The listing builds one solid part. Answer for the finished solid, in the listing's coordinates (mm). A direction names the side the tool comes from. Round coordinates to 2 decimals unless told otherwise and drop trailing zeros. Order: outer loops, then holes, each group sorted by start corner. A loop starts at its lowest first (then second) coordinate and runs counter-clockwise, first axis right, second up. Notation, with made-up numbers: (9.25, 71.25) - (21.25, 71.25) arc R11 cw to (21.25, 77.25) - close; hole circle Ø11 at (9, 48.25). An arc over 180 degrees is marked (long way). Use CSV: the item, a comma, the result in double quotes. Start each with the question number.
Item 1: Determine the mould class of faces 6 (the flat face through (0, 5, 68)), 7 (the cylindrical face through (9.87, 27.62, 43.83)), 8 (the flat face through (13.05, 24, 51)), 9 (the flat face through (-0.183, 19.859, 57.263)) for opening direction Y: +Y half, -Y half, draft (parallel to the pull), parting line (faces both ways), or undercut.
Item 2: Find section A-A, the plane x = -1. Give the vertices of the cut face in (y, z).
Item 3: Flat-ended cylindrical pins translate along their axes: P1, Ø1, axis at x = -12, z = 64.5, coming from the +Y side; P2, Ø4, axis at x = 1.5, z = 68.5, coming from the -Y side; P3, Ø6, axis at x = 9.5, y = 28.5, coming from the +Z side. Find the tip coordinate at first contact, or state that the pin passes through.
Item 4: For faces 1 (the flat face through (-20, 0, 65)), 2 (the flat face through (-0.183, 27.359, 44.273)), 3 (the flat face through (0.41, 26.28, 43.1)), 4 (the cylindrical face through (9.59, 17.09, 62.06)), 5 (the flat face through (-10, 2, 68)), determine the directions among +Z, -Z, +X, -X, +Y, -Y from which every point of the face is accessible in a straight line to the end or side of a thin tool.
Item 5: Find section D-D, the plane x = -16. Give the vertices of the cut face in (y, z), plus the area to 3 significant figures.
Item 6: Find section B-B, the plane y = 23.5. Give the vertices of the cut face in (x, z), plus the area to 3 significant figures.
Item 7: Find section C-C, the plane z = 54.5. Give the vertices of the cut face in (x, y), plus the area to 3 significant figures.
Item 8: Straight lines are drawn through the part: line 1 along Y through (x, z) = (-3, 67); line 2 along Y through (x, z) = (-4, 40); line 3 along Z through (x, y) = (13, 8). For each, find the intervals that lie inside material, in ascending order. Write a range as [from, to].
```python
from build123d import *

# Parameters (mm, degrees)
BOSS_EXTRUDE1_DEPTH     = 18
BOSS_EXTRUDE2_DEPTH     = 3
CUT_EXTRUDE3_DEPTH      = 84.253650708
CUT_EXTRUDE3_DEPTH_BACK = 84.253650708
CUT_EXTRUDE4_DEPTH      = 84.253650708
SKETCH5_R               = 1.25
SKETCH5_W               = 26.1
SKETCH5_H               = 15
CUT_EXTRUDE1_DEPTH      = 7
SKETCH6_W               = 20
SKETCH6_H               = 10
CUT_EXTRUDE2_DEPTH      = 84.253650708


with BuildPart() as part:
    # Sketch1 → Boss-Extrude1 (new body)
    with BuildSketch(Plane(origin=(0, 0, 0), x_dir=(1, 0, 0), z_dir=(0, 1, 0))):
        with BuildLine():
            Line((-29.583278322, -63.441545093), (-29.583278322, -60.115136561))
            ThreePointArc((-29.583278322, -60.115136561), (0, -67), (29.583278322, -60.115136561))
            Line((29.583278322, -60.115136561), (29.583278322, -63.441545093))
            ThreePointArc((29.583278322, -63.441545093), (0, -70), (-29.583278322, -63.441545093))
        make_face()
    extrude(amount=BOSS_EXTRUDE1_DEPTH)

    # Sketch3 → Boss-Extrude2 (add)
    with BuildSketch(Plane(origin=(0, 40.970994853, 23.654614907), x_dir=(-1, 0, 0), z_dir=(-1.9937140685199517e-15, -0.8660254037844395, -0.49999999999999856))):
        Polygon((29.583278322, -45.941989705), (29.583278322, -13.941989705), (-29.583278322, -13.941989705), (-29.583278322, -45.941989705), (-29.583278322, -53.515041118), (29.583278322, -53.515041118), align=None)
    extrude(amount=BOSS_EXTRUDE2_DEPTH)

    # Sketch7 → Cut-Extrude3 (cut, two sides: drawn at the far end of the back side and taken through both)
    with BuildSketch(Plane(origin=(0, 0, 0), x_dir=(0, 0, -1), z_dir=(1, 0, 0)).offset(-CUT_EXTRUDE3_DEPTH_BACK)):
        Polygon((-70, 14.213474294), (-63.441545093, 18), (-70, 18), align=None)
    extrude(amount=CUT_EXTRUDE3_DEPTH + CUT_EXTRUDE3_DEPTH_BACK, mode=Mode.SUBTRACT)

    # Sketch8 → Cut-Extrude4 (cut, through all)
    with BuildSketch(Plane.XZ):
        with BuildLine():
            Line((-29.583278322, 63.441545093), (-29.583278322, 71.549825609))
            Line((-29.583278322, 71.549825609), (29.583278322, 71.549825609))
            Line((29.583278322, 71.549825609), (29.583278322, 63.441545093))
            ThreePointArc((29.583278322, 63.441545093), (0, 70), (-29.583278322, 63.441545093))
        make_face()
    extrude(amount=-CUT_EXTRUDE4_DEPTH, mode=Mode.SUBTRACT)

    # Sketch5 → Cut-Extrude1 (cut)
    with BuildSketch(Plane(origin=(0, 40.970994853, 23.654614907), x_dir=(1, 0, 0), z_dir=(2.0433685445882858e-15, 0.8660254037844395, 0.49999999999999845))):
        with Locations(Location((-10.35, -22.991989705, 0), (0, 0, 270))):
            Circle(SKETCH5_R)
        with Locations(Location((10.35, -22.991989705, 0), (0, 0, 270))):
            Circle(SKETCH5_R)
        with Locations(Location((10.35, -46.191989705, 0), (0, 0, 270))):
            Circle(SKETCH5_R)
        with Locations(Location((-10.35, -46.191989705, 0), (0, 0, 270))):
            Circle(SKETCH5_R)
        with Locations((0, -32.161989705)):
            Rectangle(SKETCH5_W, SKETCH5_H)
    extrude(amount=-CUT_EXTRUDE1_DEPTH, mode=Mode.SUBTRACT)

    # Sketch6 → Cut-Extrude2 (cut, through all)
    with BuildSketch(Plane.XY):
        Rectangle(SKETCH6_W, SKETCH6_H)
    extrude(amount=CUT_EXTRUDE2_DEPTH, mode=Mode.SUBTRACT)


solid = part.part
```
Worked out:
1,face 6,"-Y half"
1,face 7,"undercut"
1,face 8,"draft"
1,face 9,"+Y half"
2,outline,"(5, 66.99) - (12.49, 66.99) - (18.54, 56.5) - (21.14, 58) - (14.22, 69.99) - (5, 69.99) - close; (26.04, 43.51) - (31.4, 34.23) - (34, 35.73) - (28.64, 45.01) - close"
3,P1,"stops at y = 17.68"
3,P2,"stops at y = 5"
3,P3,"stops at z = 45.01"
4,face 1,"+Z, -Z, +X, -X, -Y"
4,face 2,"+Z, -Y"
4,face 3,"-Z, -Y"
4,face 4,"none"
4,face 5,"+Z, -Z, -Y"
5,outline,"(0, 65.06) - (13.6, 65.06) - (31.4, 34.23) - (34, 35.73) - (15.28, 68.15) - (0, 68.15) - close"
5,area,"154 mm²"
6,outline,"(-29.58, 47.92) - (-13.05, 47.92) - (-13.05, 53.92) - (-29.58, 53.92) - close; (13.05, 47.92) - (29.58, 47.92) - (29.58, 53.92) - (13.05, 53.92) - close"
6,area,"198 mm²"
7,outline,"(-29.58, 19.7) - (-13.05, 19.7) - (-13.05, 23.16) - (-29.58, 23.16) - close; (13.05, 19.7) - (29.58, 19.7) - (29.58, 23.16) - (13.05, 23.16) - close"
7,area,"115 mm²"
8,line 1,"y = [5, 15.95]"
8,line 2,"y = [28.07, 31.53]"
8,line 3,"z = [65.73, 68.78]"
